Input: dimensioned drawing with shaded views. Units: mm. Origin: part minimum x, y, z. Round coordinates to 2 decimals unless told otherwise and drop trailing zeros. Loops run counter-clockwise (first coordinate to the right, second up) from the corner with the lowest first, then second, coordinate; pieces in that order, holes last. Notation, with made-up numbers: M 30,55.25 L 43,55.25 A38 ccw 43,93.25 Z; hole C 77.5,51 d3. An arc over 180 degrees is marked long. Put each result on its own line as item: value. Start each with the question number.
1) Section B-B on y = 20. Output: boundary loops of the cut face in (x, z).
2) Section A-A on x = 2.5. Output: boundary loops of the cut face in (y, z).
3) Section D-D on x = 17. Output: boundary loops of the cut face in (y, z), plus the area to 3 significant figures.
4) Section C-C on z = 48.5. Output: boundary loops of the cut face in (x, y) (1 decimal).
5) Pin query (flat end, axial travel): pin 1 (1.4 mm diameter, centred on x = 2.5, z = 48.5, fed in from -Y); pin 2 (12.5 mm diameter, centred on x = 28.5, z = 28.5, fed in from +Y). Return the tip coordinate at first contact, or that it passes through.
6) Line query: probe 1 along X at (y, z) = (25, 48.5) (1 decimal); probe 2 along Z at (x, y) = (2, 22) (1 decimal); probe 3 along Y at (x, z) = (10.5, 19). Output: solid intervals per line, ascending.
7) Draft query along X for the marked faces 1, 2, 3 and 4. Return one class per face: +X half, -X half, draft (parallel to the pull), parting line (faces both ways), or undercut.
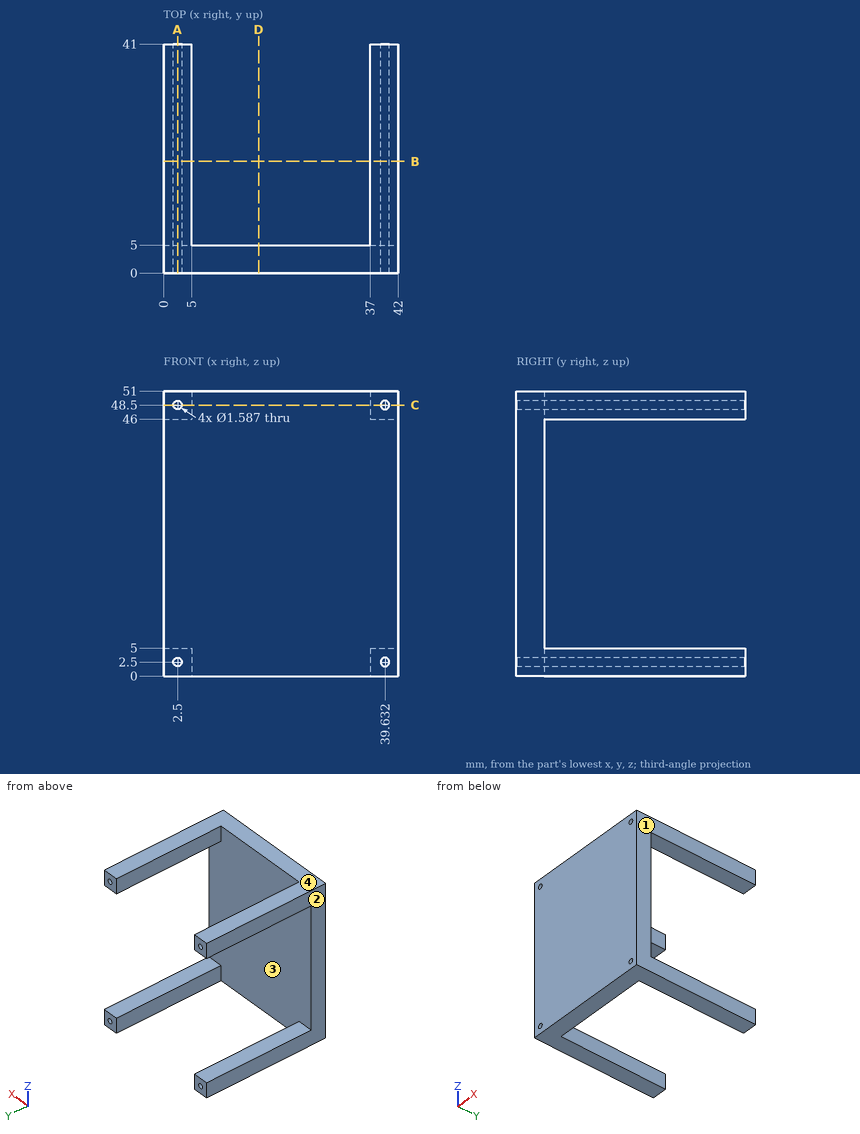
Geometry results:
1. outline: M 0,0 L 5,0 L 5,5 L 0,5 Z; M 0,46 L 5,46 L 5,51 L 0,51 Z; M 37,0 L 42,0 L 42,5 L 37,5 Z; M 37,46 L 42,46 L 42,51 L 37,51 Z; hole C 2.5,2.5 d1.59; hole C 2.5,48.5 d1.59; hole C 39.63,2.5 d1.59; hole C 39.63,48.5 d1.59
2. outline: M 0,0 L 41,0 L 41,1.71 L 0,1.71 Z; M 0,3.29 L 41,3.29 L 41,5 L 5,5 L 5,46 L 41,46 L 41,47.71 L 0,47.71 Z; M 0,49.29 L 41,49.29 L 41,51 L 0,51 Z
3. outline: M 0,0 L 5,0 L 5,51 L 0,51 Z
3. area: 255 mm²
4. outline: M 0,0 L 1.7,0 L 1.7,41 L 0,41 Z; M 3.3,0 L 38.8,0 L 38.8,41 L 37,41 L 37,5 L 5,5 L 5,41 L 3.3,41 Z; M 40.4,0 L 42,0 L 42,41 L 40.4,41 Z
5. pin 1: passes through
5. pin 2: stops at y = 5
6. probe 1: x = 0 to 1.7, 3.3 to 5, 37 to 38.8, 40.4 to 42
6. probe 2: z = 0 to 1.9, 3.1 to 5, 46 to 47.9, 49.1 to 51
6. probe 3: y = 0 to 5
7. face 1: +X half
7. face 2: -X half
7. face 3: undercut
7. face 4: draft
